Verification items for the finished model (mm, model axes). Give positions to 0.01 mm unless a question says otherwise; leave off trailing zeros. Order: outer loops, then holes, each group sorted by start corner. A loop starts at its lowest first (then second) coordinate and runs counter-clockwise, first axis right, second up. Notation, with made-up numbers: (61, 1.5) -> (103, 1.5) arc R11 cw to (103, 14.5) -> close; hole circle Ø8 at (82, 59.5). An arc over 180 degrees is marked (long way). Return JSON: item names as keys, results as strings. Group by question number.
(1) Release check for a two-part mould opening along Z. For faces 1 (the face through (457.2, -16, 272)), 2 (the face through (60.697, -15.653, 51.516)), 3 (the face through (347, -16, 304.8)), 4 (the face through (202.27, -16.1, 1.88)) record: pulls with the +Z half, pulls with the -Z half, needs draft (parallel to the pull), parting line crosses it, or undercut.
(2) Cross-section at D-D on x = 156. Enter the section's corners in (y, z), then the cut area to 3 significant figures.
(3) Cross-section at A-A on x = 228.6. Enter the section's corners in (y, z).
(4) Thickness scan on line 1 along Z through (x, y) = (228, -20); line 2 along Z through (x, y) = (61, -11); line 3 along X through (y, z) = (-6.5, 145.5). Record the ranges inside material, lowest first.
(5) Depth check by flat-ended pin: pin 1 Ø7.5 at (x, z) = (393.573, 247.65) entering from +Y; pin 2 Ø5 at (x, y) = (127, -22.5) entering from +Z; pin 3 Ø4 at (x, y) = (171.5, -11.5) entering from +Z; pin 4 Ø2 at (y, z) = (-11, 111) entering from -X. Enter the tip coordinate at first touch or a pass-through.
(6) Cross-section at B-B on z = 152.4. Enter the section's corners in (x, y).
(7) Cross-section at C-C on y = -24. Enter the section's corners in (x, z), then the cut area to 3 significant figures.
from build123d import *

# Parameters (mm, degrees)
F0_W     = 457.2
F0_H     = 304.8
F1_DEPTH = 31.75
F2_SIZE2 = 254
F2_SIZE  = 254
F3_R     = 25.4
F5_D     = 12.7
F8_D     = 25.4


with BuildPart() as f1:
    # F0 (on Front) → F1 (new body)
    with BuildSketch(Plane.XZ):
        with Locations((228.6, 152.4)):
            Rectangle(F0_W, F0_H)
    extrude(amount=F1_DEPTH)

    # F2
    f2_edges = [f1.edges().sort_by_distance(p)[0] for p in [
        (0, -15.875, 304.8),
        (457.2, -15.875, 0),
    ]]
    chamfer(f2_edges, length=F2_SIZE, length2=F2_SIZE2)

    # F3
    f3_edges = [f1.edges().sort_by_distance(p)[0] for p in [
        (0, -15.875, 50.8),
        (0, -15.875, 0),
        (203.2, -15.875, 0),
        (457.2, -15.875, 254),
        (457.2, -15.875, 304.8),
        (254, -15.875, 304.8),
    ]]
    fillet(f3_edges, radius=F3_R)

    # F5 (through all)
    with Locations(Plane.XZ.offset(31.75)):
        with Locations((63.627, 57.15), (393.573, 247.65)):
            Hole(F5_D / 2)

    # F8 (through all)
    with Locations(Plane.XZ.offset(31.75)):
        with Locations((228.6, 152.4)):
            Hole(F8_D / 2)


solid = f1.part
Verdict:
{
 "1": {"face 1": "needs draft", "face 2": "undercut", "face 3": "pulls with the +Z half", "face 4": "pulls with the -Z half"},
 "2": {"outline": "(-31.75, 0) -> (0, 0) -> (0, 206.8) -> (-31.75, 206.8) -> close", "area": "6,570 mm²"},
 "3": {"outline": "(-31.75, 25.4) -> (0, 25.4) -> (0, 139.7) -> (-31.75, 139.7) -> close; (-31.75, 165.1) -> (0, 165.1) -> (0, 279.4) -> (-31.75, 279.4) -> close"},
 "4": {"line 1": "24.8 to 139.71, 165.09 to 278.8", "line 2": "0 to 51.37, 62.93 to 111.8", "line 3": "94.7 to 217.94, 239.26 to 348.7"},
 "5": {"pin 1": "through", "pin 2": "z = 180.3", "pin 3": "z = 224.3", "pin 4": "x = 59.2"},
 "6": {"outline": "(101.6, -31.75) -> (215.9, -31.75) -> (215.9, 0) -> (101.6, 0) -> close; (241.3, -31.75) -> (355.6, -31.75) -> (355.6, 0) -> (241.3, 0) -> close"},
 "7": {"outline": "(0, 25.4) arc R25.4 ccw to (25.4, 0) -> (192.68, 0) arc R25.4 ccw to (210.64, 7.44) -> (449.76, 246.56) arc R25.4 ccw to (457.2, 264.52) -> (457.2, 279.4) arc R25.4 ccw to (431.8, 304.8) -> (264.52, 304.8) arc R25.4 ccw to (246.56, 297.36) -> (7.44, 58.24) arc R25.4 ccw to (0, 40.28) -> close; hole circle Ø12.7 at (63.63, 57.15); hole circle Ø25.4 at (228.6, 152.4); hole circle Ø12.7 at (393.57, 247.65)", "area": "73,700 mm²"}
}
